CAD build for the part. Positions are in the model's coordinates, mm. Coordinates: 2 decimals unless noted, no trailing zeros. Order: outer loops, then holes, each group sorted by start corner. A loop starts at its lowest first (then second) coordinate and runs counter-clockwise, first axis right, second up. Notation, with made-up numbers: (22, 68) - (37, 68) arc R16 cw to (37, 80) - close; hole circle Ø5 at (47, -32.75). An arc over 180 degrees is marked (long way). Use one line per item in the form item = value.
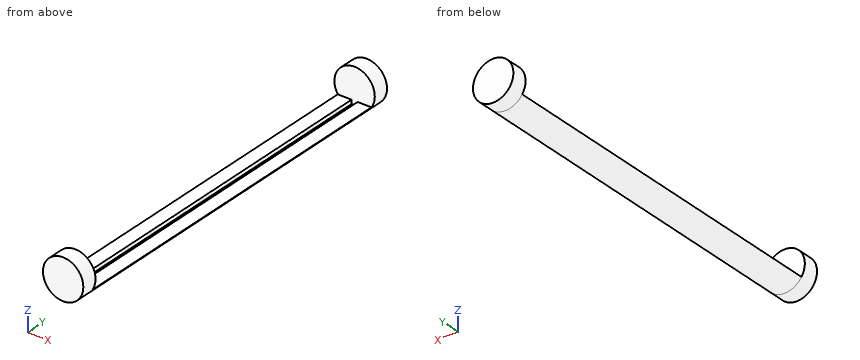
```python
from build123d import *

# Parameters (mm, degrees)
F1_DEPTH = 114.3
F2_R     = 12.7
F3_DEPTH = 10
F4_W     = 3.81
F4_H     = 2.5
F5_DEPTH = 114.3


with BuildPart() as f1:
    # F0 (on Front) → F1 (new body)
    with BuildSketch(Plane.XZ):
        with BuildLine():
            Line((10.596698, -7), (-10.596698, -7))
            ThreePointArc((-10.596698, -7), (0, -12.7), (10.596698, -7))
        make_face()
    extrude(amount=F1_DEPTH)

    # F2 (on face) → F3 (join)
    with BuildSketch(Plane.XZ.offset(114.3)):
        Circle(F2_R)
    extrude(amount=F3_DEPTH)

    # F4 (on face) → F5 (cut)
    with BuildSketch(Plane(origin=(0, 0, 0), x_dir=(-1, 0, 0), z_dir=(0, 1, 0))):
        with Locations((0, -8.25)):
            Rectangle(F4_W, F4_H)
    extrude(amount=-F5_DEPTH, mode=Mode.SUBTRACT)

    # F6: F1 across face


with BuildPart() as f1_1:
    add(f1.part)
    add(f1.part.mirror(Plane(origin=(0, 0, -9.466797), x_dir=(1, 0, 0), z_dir=(0, 1, 0))))


solid = f1_1.part
```
Item 1: Drill centre lines: line 1 (Y direction, x = 0.25, z = 0); line 2 (Z direction, x = -10.25, y = -104); line 3 (Z direction, x = -5.5, y = 33). Where is each one in solid material? Low to high. Write a range as [from, to].
Derived:
line_1 = [-124.3, -114.3], [114.3, 124.3]
line_2 = [-7.5, -7]
line_3 = [-11.45, -7]
Item 2: Cut at B-B, the plane y = -69. Write the cut outline in (x, z) (3 decimals).
Derived:
outline = (-10.597, -7) arc R12.7 ccw to (10.597, -7) - (1.905, -7) - (1.905, -9.5) - (-1.905, -9.5) - (-1.905, -7) - close
Item 3: Drop flat-ended pins along their axis: pin 1 (3 mm diameter, centred on y = 48, z = -8, fed in from +X); pin 2 (7 mm diameter, centred on x = 8, y = -13.5, fed in from +Z); pin 3 (1.9 mm diameter, centred on x = -0.5, y = 53.5, fed in from +Z). Give the stop position or say it passes through.
Derived:
pin_1 = 10.6
pin_2 = -7
pin_3 = -9.5
Item 4: Cut at C-C, the plane x = 4.75. Write the cut outline in (y, z).
Derived:
outline = (-124.3, -11.78) - (124.3, -11.78) - (124.3, 11.78) - (114.3, 11.78) - (114.3, -7) - (-114.3, -7) - (-114.3, 11.78) - (-124.3, 11.78) - close
Item 5: Cut at A-A, the plane z = 0. Write the cut outline in (x, y).
Derived:
outline = (-12.7, -124.3) - (12.7, -124.3) - (12.7, -114.3) - (-12.7, -114.3) - close; (-12.7, 114.3) - (12.7, 114.3) - (12.7, 124.3) - (-12.7, 124.3) - close
